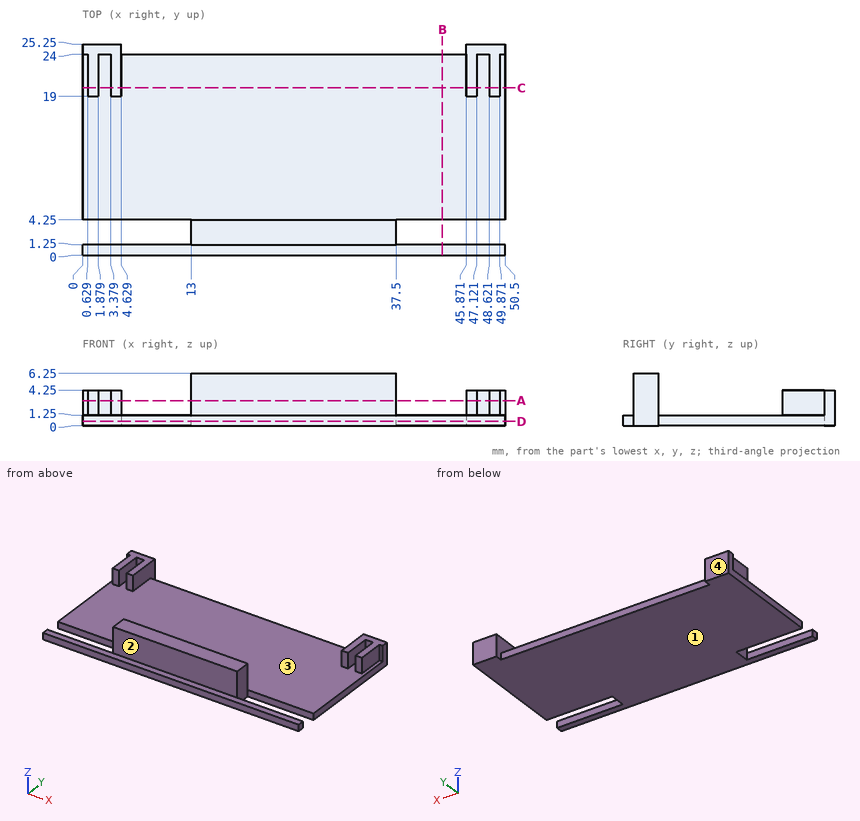
Print and shaded views of the part. All mm, measured from the part's lowest x, y and z. A direction names the side the tool comes from. Give positions to 0.01 mm unless a question says otherwise; leave off trailing zeros. Order: outer loops, then holes, each group sorted by start corner. A loop starts at its lowest first (then second) coordinate and runs counter-clockwise, first axis right, second up. Notation, with made-up numbers: (10, 72.25) - (62, 72.25) arc R18 cw to (62, 104.25) - close; hole circle Ø1 at (49, 32.5). An arc over 180 degrees is marked (long way). One line per item, written item: value.
Item 1: Slice it at B-B (x = 43). List the corners of the cut face in (y, z).
Response values:
outline: (0, 0) - (1.25, 0) - (1.25, 1.25) - (0, 1.25) - close; (4.25, 0) - (24, 0) - (24, 1.25) - (4.25, 1.25) - close
Item 2: Slice it at D-D (z = 0.5). List the corners of the cut face in (x, y), then the cut area to 3 significant figures.
Response values:
outline: (0, 0) - (50.5, 0) - (50.5, 1.25) - (37.5, 1.25) - (37.5, 4.25) - (50.5, 4.25) - (50.5, 25.25) - (45.87, 25.25) - (45.87, 24) - (4.63, 24) - (4.63, 25.25) - (0, 25.25) - (0, 4.25) - (13, 4.25) - (13, 1.25) - (0, 1.25) - close
area: 1,150 mm2
Item 3: Two-plate mould, pull along X, no slides. Class the marked faces 3 and 4: released by +X, released by -X, zero draft, split by the parting line, or undercut.
Response values:
face 3: undercut
face 4: zero draft
Item 4: Slice it at C-C (y = 20). List the corners of the cut face in (x, z).
Response values:
outline: (0, 0) - (50.5, 0) - (50.5, 1.25) - (49.87, 1.25) - (49.87, 4.25) - (48.62, 4.25) - (48.62, 1.25) - (47.12, 1.25) - (47.12, 4.25) - (45.87, 4.25) - (45.87, 1.25) - (4.63, 1.25) - (4.63, 4.25) - (3.38, 4.25) - (3.38, 1.25) - (1.88, 1.25) - (1.88, 4.25) - (0.63, 4.25) - (0.63, 1.25) - (0, 1.25) - close
Item 5: Wall check: line 1 (X direction, y = 20.5, z = 3.75); line 2 (Y direction, x = 42, z = 0.5); line 3 (Y direction, x = 21, z = 1.5). Give the ranges that are in metal, low to high.
Response values:
line 1: 0.63 to 1.88, 3.38 to 4.63, 45.87 to 47.12, 48.62 to 49.87
line 2: 0 to 1.25, 4.25 to 24
line 3: 1.25 to 4.25
Item 6: Pin check, flat tips, straight feed: pin 1 Ø2 at (x, y) = (8.5, 17.5) entering from -Z; pin 2 Ø1.4 at (x, z) = (43, 0.5) entering from +Y; pin 3 Ø2.5 at (x, z) = (27, 4) entering from -Y; pin 4 Ø1.3 at (y, z) = (23, 3) entering from -X. Stop position of each tip, or through.
Response values:
pin 1: z = 0
pin 2: y = 24
pin 3: y = 1.25
pin 4: x = 0.63
Item 7: Tool access for the marked faces 1 and 2: list every direction of +Z, -Z, +X, -X, +Y, -Y with a clear straight run to the whole face (end or side of a thin tool).
Response values:
face 1: -Z, +X, -X, +Y, -Y
face 2: +Z, +X, -X, -Y
Item 8: Slice it at A-A (z = 3). List the corners of the cut face in (x, y), then the cut area to 3 significant figures.
Response values:
outline: (0, 24) - (0.63, 24) - (0.63, 19) - (1.88, 19) - (1.88, 24) - (3.38, 24) - (3.38, 19) - (4.63, 19) - (4.63, 25.25) - (0, 25.25) - close; (13, 1.25) - (37.5, 1.25) - (37.5, 4.25) - (13, 4.25) - close; (45.87, 19) - (47.12, 19) - (47.12, 24) - (48.62, 24) - (48.62, 19) - (49.87, 19) - (49.87, 24) - (50.5, 24) - (50.5, 25.25) - (45.87, 25.25) - close
area: 110 mm2
